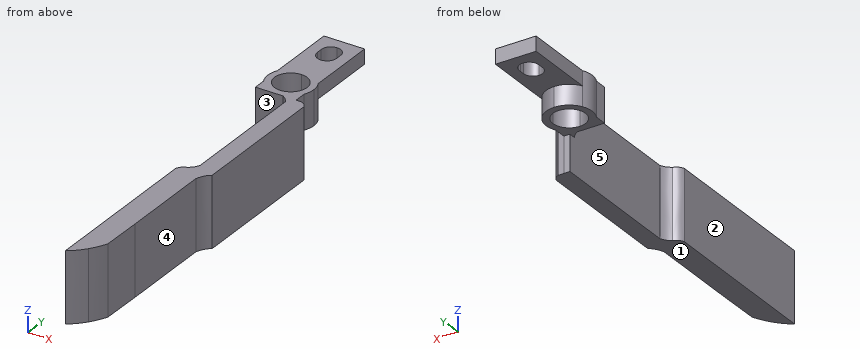
from build123d import *

# Parameters (mm, degrees)
F1_DEPTH = 5.9
F2_DEPTH = 2.5
F3_DEPTH = 12
F4_DEPTH = 12


with BuildPart() as f1:
    # F0 (on Top) → F1 (new body)
    with BuildSketch(Plane.XY):
        with BuildLine():
            Line((0, 2.1001712409), (0, 0))
            Line((0, 0), (1.025, 0))
            Line((1.025, 0), (1.025, 0.8585484677))
            ThreePointArc((1.025, 0.8585484677), (0.4481513041, 1.426237912), (0, 2.1001712409))
        make_face()
        with BuildLine():
            Line((1.025, 0.8585484677), (1.025, 0))
            Line((1.025, 0), (3.475, 0))
            ThreePointArc((3.475, 0), (2.1769624937, 0.2208504846), (1.025, 0.8585484677))
        make_face()
        with BuildLine():
            ThreePointArc((0, 5.7498287591), (-0.45, 3.925), (0, 2.1001712409))
            Line((0, 2.1001712409), (0, 5.7498287591))
        make_face()
        with BuildLine():
            Line((0, 5.7498287591), (0, 2.1001712409))
            ThreePointArc((0, 2.1001712409), (0.4481513041, 1.426237912), (1.025, 0.8585484677))
            ThreePointArc((1.025, 0.8585484677), (2.1769624937, 0.2208504846), (3.475, 0))
            Line((3.475, 0), (3.475, 1.15))
            ThreePointArc((3.475, 1.15), (0.7, 3.925), (3.475, 6.7))
            Line((3.475, 6.7), (3.475, 6.8908035755))
            Line((3.475, 6.8908035755), (3.475, 7.85))
            ThreePointArc((3.475, 7.85), (1.4448310267, 7.2841723593), (0, 5.7498287591))
        make_face()
        with BuildLine():
            ThreePointArc((5.925, 0.8585484677), (4.7730375063, 0.2208504846), (3.475, 0))
            Line((3.475, 0), (4.7, 0))
            Line((4.7, 0), (5.925, 0))
            Line((5.925, 0), (5.925, 0.8585484677))
        make_face()
        with BuildLine():
            Line((3.475, 1.15), (3.475, 0))
            ThreePointArc((3.475, 0), (4.7730375063, 0.2208504846), (5.925, 0.8585484677))
            ThreePointArc((5.925, 0.8585484677), (6.5018486959, 1.426237912), (6.95, 2.1001712409))
            Line((6.95, 2.1001712409), (6.95, 5.7498287591))
            ThreePointArc((6.95, 5.7498287591), (5.5051689733, 7.2841723593), (3.475, 7.85))
            Line((3.475, 7.85), (3.475, 6.8908035755))
            Line((3.475, 6.8908035755), (3.475, 6.7))
            ThreePointArc((3.475, 6.7), (5.4372213178, 5.8872213178), (6.25, 3.925))
            ThreePointArc((6.25, 3.925), (5.4372213178, 1.9627786822), (3.475, 1.15))
        make_face()
        with BuildLine():
            Line((5.925, 0), (4.7, 0))
            add(Edge.make_bspline(
                [(4.7, 0), (5.2537494339, -0.3164176305), (5.6369397789, -0.7196032093), (5.925, -1.225)],
                knots=[0, 0, 0, 0, 1.7324116139, 1.7324116139, 1.7324116139, 1.7324116139], degree=3))
            Line((5.925, -1.225), (5.925, -0.079424061))
            Line((5.925, -0.079424061), (5.925, 0))
        make_face()
        with BuildLine():
            ThreePointArc((6.95, 2.1001712409), (6.5018486959, 1.426237912), (5.925, 0.8585484677))
            Line((5.925, 0.8585484677), (5.925, 0))
            Line((5.925, 0), (6.95, 0))
            Line((6.95, 0), (6.95, 0.75))
            Line((6.95, 0.75), (6.95, 1.44))
            Line((6.95, 1.44), (6.95, 1.5))
            Line((6.95, 1.5), (6.95, 2.1001712409))
        make_face()
        with BuildLine():
            Line((6.95, 5.7498287591), (6.95, 2.1001712409))
            ThreePointArc((6.95, 2.1001712409), (7.2858398025, 2.9852526935), (7.4, 3.925))
            ThreePointArc((7.4, 3.925), (7.2858398025, 4.8647473065), (6.95, 5.7498287591))
        make_face()
    extrude(amount=-F1_DEPTH)

    # F0 (on Top) → F2 (join)
    with BuildSketch(Plane.XY):
        with BuildLine():
            Line((0, 7.85), (0, 5.7498287591))
            ThreePointArc((0, 5.7498287591), (1.4448310267, 7.2841723593), (3.475, 7.85))
            ThreePointArc((3.475, 7.85), (5.5051689733, 7.2841723593), (6.95, 5.7498287591))
            Line((6.95, 5.7498287591), (6.95, 17.9))
            Line((6.95, 17.9), (3.475, 17.9))
            Line((3.475, 17.9), (0, 17.9))
            Line((0, 17.9), (0, 7.85))
        make_face()
        with BuildLine():
            ThreePointArc((1.8276640256, 14.3833613398), (2.3042302705, 15.55900427), (3.475, 16.0474200003))
            ThreePointArc((3.475, 16.0474200003), (4.5253988967, 15.6691157612), (5.0933824344, 14.7079463483))
            Line((5.0933824344, 14.7079463483), (5.1024433757, 14.1442252627))
            Line((5.1024433757, 14.1442252627), (5.113982201, 13.4263440945))
            ThreePointArc((5.113982201, 13.4263440945), (5.1141409801, 13.4131724726), (5.1141939076, 13.4))
            ThreePointArc((5.1141939076, 13.4), (4.6340851277, 12.2409148723), (3.475, 11.7608060924))
            ThreePointArc((3.475, 11.7608060924), (2.2942628451, 12.2629791393), (1.8369719791, 13.4618131819))
            Line((1.8369719791, 13.4618131819), (1.8276640256, 14.3833613398))
        make_face(mode=Mode.SUBTRACT)
    extrude(amount=-F2_DEPTH)

    # F0 (on Top) → F3 (join)
    with BuildSketch(Plane.XY):
        with BuildLine():
            Line((6.95, 0), (5.925, 0))
            Line((5.925, 0), (5.925, -0.079424061))
            Line((5.925, -0.079424061), (5.925, -1.225))
            Line((5.925, -1.225), (5.925, -21.3844068348))
            Line((5.925, -21.3844068348), (5.925, -22.55))
            Line((5.925, -22.55), (5.925, -22.9875))
            Line((5.925, -22.9875), (5.925, -23.5205553472))
            Line((5.925, -23.5205553472), (5.925, -25))
            Line((5.925, -25), (7.525, -25))
            Line((7.525, -25), (8.9492390995, -25))
            Line((8.9492390995, -25), (8.9492390995, -0.9913714603))
            add(Edge.make_bspline(
                [(7.9496195498, -0.0275818011), (8.4295123816, -0.2455351059), (8.7658986449, -0.6068330258), (8.9492390995, -0.9913714603)],
                knots=[0, 0, 0, 0, 1.3885711186, 1.3885711186, 1.3885711186, 1.3885711186], degree=3))
            Line((7.9496195498, -0.0275818011), (6.95, 0))
        make_face()
        with BuildLine():
            add(Edge.make_bspline(
                [(4.7, -25), (4.0586842224, -25.2618398517), (3.6450892221, -25.6055109203), (3.475, -26.225)],
                knots=[0, 0, 0, 0, 1.7324116139, 1.7324116139, 1.7324116139, 1.7324116139], degree=3))
            Line((3.475, -26.225), (3.475, -48.775))
            Line((3.475, -48.775), (3.475, -50))
            Line((3.475, -50), (5.925, -50))
            Line((5.925, -50), (5.925, -47.55))
            Line((5.925, -47.55), (5.925, -43))
            Line((5.925, -43), (5.925, -28.903))
            Line((5.925, -28.903), (5.925, -26.9515))
            Line((5.925, -26.9515), (5.925, -25))
            Line((5.925, -25), (4.7, -25))
        make_face()
        with BuildLine():
            add(Edge.make_bspline(
                [(4.7, -25), (5.3314492106, -24.6048551053), (5.6424522772, -24.1878218949), (5.925, -23.5205553472)],
                knots=[0, 0, 0, 0, 1.9207762703, 1.9207762703, 1.9207762703, 1.9207762703], degree=3))
            Line((4.7, -25), (5.925, -25))
            Line((5.925, -25), (5.925, -23.5205553472))
        make_face()
        Polygon((7.525, -25), (5.925, -25), (5.925, -26.9515), (5.925, -28.903), (5.925, -43), (7.525, -43), (7.525, -27.1006729454), align=None)
        with BuildLine():
            add(Edge.make_bspline(
                [(8.9492390995, -25), (8.2447035238, -25.5232192576), (7.9111177474, -26.03264153), (7.525, -27.1006729454)],
                knots=[0, 0, 0, 0, 2.5379684466, 2.5379684466, 2.5379684466, 2.5379684466], degree=3))
            Line((8.9492390995, -25), (7.525, -25))
            Line((7.525, -25), (7.525, -27.1006729454))
        make_face()
        with BuildLine():
            Line((5.925, -50), (3.475, -50))
            Line((3.475, -50), (3.475, -55))
            add(Edge.make_bspline(
                [(3.475, -55), (4.512583722, -54.3078648135), (5.2908616095, -53.5264365704), (5.925, -52.6706067544)],
                knots=[0, 0, 0, 0, 3.2551675464, 3.2551675464, 3.2551675464, 3.2551675464], degree=3))
            Line((5.925, -52.6706067544), (5.925, -52.0125))
            Line((5.925, -52.0125), (5.925, -50))
        make_face()
        with BuildLine():
            Line((7.4536274492, -50.0155514561), (5.925, -50))
            Line((5.925, -50), (5.925, -52.0125))
            Line((5.925, -52.0125), (5.925, -52.6706067544))
            add(Edge.make_bspline(
                [(5.925, -52.6706067544), (6.5332867434, -51.8496661845), (7.0089465882, -50.9602665865), (7.4536274492, -50.0155514561)],
                knots=[3.2551675464, 3.2551675464, 3.2551675464, 3.2551675464, 6.3776330772, 6.3776330772, 6.3776330772, 6.3776330772], degree=3))
        make_face()
        Polygon((5.925, -47.55), (5.925, -50), (7.4537856616, -50), (7.525, -43), (5.925, -43), align=None)
    extrude(amount=-F3_DEPTH)

    # F0 (on Top) → F4 (join)
    with BuildSketch(Plane.XY):
        Polygon((7.4537856616, -50), (5.925, -50), (7.4536274492, -50.0155514561), align=None)
    extrude(amount=-F4_DEPTH)


solid = f1.part
Source: CAD feature listing. Evaluate the final solid. Frame: model axes, mm. Face numbers are marked on the shaded views. A direction names the side the tool comes from. Round coordinates to 2 decimals unless told otherwise and drop trailing zeros. Order: outer loops, then holes, each group sorted by start corner. A loop starts at its lowest first (then second) coordinate and runs counter-clockwise, first axis right, second up. Notation, with made-up numbers: (83.5, 85.5) - (118.5, 85.5) arc R16 cw to (118.5, 114.5) - close; hole circle Ø10 at (-29, 19.25). An arc over 180 degrees is marked (long way). Use a Markdown table: item, result. Add a question column.
1. First-contact query: pin 1 (0.8 mm diameter, centred on y = 13, z = -1, fed in from +X); pin 2 (1 mm diameter, centred on x = 5.5, z = -10.5, fed in from -Y); pin 3 (1.7 mm diameter, centred on y = 0.5, z = -2, fed in from -X). Flat tips, straight axial feed; report the tip coordinate or a pass-through.
2. Section query B-B (y = -42). Return the cut outline in (x, z) (3 decimals), then the cut area to 3 significant figures.
3. Line query: probe 1 along X at (y, z) = (-13.5, -4) (3 decimals); probe 2 along Y at (x, z) = (0.5, -1.5); probe 3 along Z at (x, y) = (6, 7). Output: solid intervals per line, ascending.
4. Set-up query: the marked faces 1, 2 and 3. Return all of +Z, -Z, +X, -X, +Y, -Y with unobstructed straight access to the full face (end or side cutting, diameter ignored); none if empty.
5. Section query A-A (y = -3.5). Return the cut outline in (x, z) (3 decimals), then the cut area to 3 significant figures.
6. Mould query, pull axis Y, two halves, no side actions, for the marked faces 4 and 5. Classes: +Y half, -Y half, draft (parallel to the pull), parting line (faces both ways), or undercut.
Derived:
| question | item | result |
|---|---|---|
| 1 | pin 1 | x = 6.95 |
| 1 | pin 2 | y = -53.75 |
| 1 | pin 3 | x = 0 |
| 2 | outline | (3.475, -12) - (7.525, -12) - (7.525, 0) - (3.475, 0) - close |
| 2 | area | 48.6 mm2 |
| 3 | probe 1 | 5.925 to 8.949 |
| 3 | probe 2 | 0 to 17.9 |
| 3 | probe 3 | -2.5 to 0 |
| 4 | face 1 | -Z, +X, -X, +Y, -Y |
| 4 | face 2 | +Z, -Z, -X, -Y |
| 4 | face 3 | +Z, -Z, -X |
| 5 | outline | (5.925, -12) - (8.949, -12) - (8.949, 0) - (5.925, 0) - close |
| 5 | area | 36.3 mm2 |
| 6 | face 4 | draft |
| 6 | face 5 | undercut |
